Autodesk Inventor part; units mm, degrees
ref_plane "YZ Plane" through (0, 0, 0) normal (1, 0, 0) x (0, 1, 0)
ref_plane "XZ Plane" through (0, 0, 0) normal (0, 1, 0) x (-1, 0, 0)
ref_plane "XY Plane" through (0, 0, 0) normal (0, 0, 1) x (1, 0, 0)
sketch "Sketch1" plane through (0, 0, 0) normal (0, 1, 0) x (-1, 0, 0)
  line L0 (140, 210) -> (-140, 210)
  line L1 (-140, 210) -> (-140, -210)
  line L2 (-140, -210) -> (140, -210)
  line L3 (140, -210) -> (140, 210)
  line L4 (140, 210) -> (-140, -210) construction
  line L5 (-140, 210) -> (140, -210) construction
  point P0 (0, 0)
  dimension "d0" = 280
  dimension "d1" = 420
extrude "Extrusion1" add sketch "Sketch1" along normal blind 6
sketch "Sketch2" plane through (0, 6, 0) normal (0, 1, 0) x (1, 0, 0)
  circle A0 centre (105, -175) radius 14
  line L0 (-140, -210) -> (140, -210)
  line L1 (140, -210) -> (140, 210)
  point P0 (0, 0)
  dimension "d4" = 28
  dimension "d5" = 35
  dimension "d6" = 35
extrude "Extrusion2" cut sketch "Sketch2" against normal blind 6
sketch "Sketch3" plane through (0, 6, 0) normal (0, 1, 0) x (1, 0, 0)
  circle A0 centre (135, -205) radius 1.75
  line L0 (-140, -210) -> (140, -210)
  line L1 (140, -210) -> (140, 210)
  circle A1 centre (75.5, -205) radius 1.75
  circle A2 centre (135, -145.5) radius 1.75
  circle A3 centre (75.5, -145.5) radius 1.75
  point P0 (0, 0)
  dimension "d15" = 3.5
  dimension "d16" = 5
  dimension "d17" = 5
  dimension "d18" = 3.5
  dimension "d19" = 5
  dimension "d20" = 59.5
  dimension "d21" = 3.5
  dimension "d22" = 5
  dimension "d23" = 59.5
  dimension "d24" = 3.5
  dimension "d25" = 59.5
  dimension "d26" = 59.5
pattern_linear "Rectangular Pattern1" count 6 spacing 70 along (0, 0, -1) count 4 spacing 70 along (-1, 0, 0) of "Extrusion2"
sketch "Sketch4" plane through (0, 6, 0) normal (0, 1, 0) x (1, 0, 0)
  line L0 (140, -210) -> (140, 210)
  line L1 (140, -25) -> (134, -25)
  line L2 (134, -25) -> (134, 25)
  line L3 (134, 25) -> (140, 25)
  line L4 (140, 25) -> (140, -25)
  line L5 (0, -210) -> (0, 210) construction
  line L6 (140, -165) -> (134, -165)
  line L7 (134, -165) -> (134, -115)
  line L8 (134, -115) -> (140, -115)
  line L9 (140, -115) -> (140, -165)
  line L10 (-140, -210) -> (140, -210)
  line L11 (140, 115) -> (134, 115)
  line L12 (134, 115) -> (134, 165)
  line L13 (134, 165) -> (140, 165)
  line L14 (140, 165) -> (140, 115)
  line L15 (140, 210) -> (-140, 210)
  line L16 (-140, -25) -> (-134, -25)
  line L17 (-134, -25) -> (-134, 25)
  line L18 (-134, 25) -> (-140, 25)
  line L19 (-140, 25) -> (-140, -25)
  line L20 (-140, -165) -> (-134, -165)
  line L21 (-134, -165) -> (-134, -115)
  line L22 (-134, -115) -> (-140, -115)
  line L23 (-140, -115) -> (-140, -165)
  line L24 (-140, 115) -> (-134, 115)
  line L25 (-134, 115) -> (-134, 165)
  line L26 (-134, 165) -> (-140, 165)
  line L27 (-140, 165) -> (-140, 115)
  line L28 (-95, -210) -> (-45, -210)
  line L29 (-45, -210) -> (-45, -204)
  line L30 (-45, -204) -> (-95, -204)
  line L31 (-95, -204) -> (-95, -210)
  line L32 (-140, 210) -> (-140, -210)
  line L33 (45, -210) -> (95, -210)
  line L34 (95, -210) -> (95, -204)
  line L35 (95, -204) -> (45, -204)
  line L36 (45, -204) -> (45, -210)
  line L37 (-140, 0) -> (140, 0) construction
  line L38 (-95, 210) -> (-45, 210)
  line L39 (-45, 210) -> (-45, 204)
  line L40 (-45, 204) -> (-95, 204)
  line L41 (-95, 204) -> (-95, 210)
  line L42 (45, 210) -> (95, 210)
  line L43 (95, 210) -> (95, 204)
  line L44 (95, 204) -> (45, 204)
  line L45 (45, 204) -> (45, 210)
  point P0 (0, 0)
  dimension "d35" = 6
  dimension "d36" = 50
  dimension "d37" = 6
  dimension "d38" = 50
  dimension "d39" = 45
  dimension "d40" = 6
  dimension "d41" = 50
  dimension "d42" = 45
  dimension "d43" = 50
  dimension "d44" = 6
  dimension "d45" = 45
  dimension "d46" = 50
  dimension "d47" = 6
  dimension "d48" = 45
extrude "Extrusion4" cut sketch "Sketch4" against normal blind 6 contours L6 L7 L8 L0 | L10 L36 L35 L34 | L1 L2 L3 L0 | L10 L31 L30 L29 | L11 L12 L13 L0 | L23 L22 L21 L20 | L43 L44 L45 L15 | L19 L18 L17 L16 | L39 L40 L41 L15 | L27 L26 L25 L24
equation "\"d17\" = d16"
equation "\"d19\" = d16"
equation "\"d22\" = d16"
equation "\"d23\" = d20"
equation "\"d25\" = d20"
equation "\"d26\" = d20"
properties part number "Base_modulos"
Read the model definition and answer for the solid it produces. Units are mm, in the model's axes. Coordinates: 2 decimals unless noted, no trailing zeros. Loops run counter-clockwise (first coordinate to the right, second up) from the corner with the lowest first, then second, coordinate; pieces in that order, holes last. Notation, with made-up numbers: (22.25, 63.25) - (70.25, 63.25) arc R37 ccw to (70.25, 102.25) - close; hole circle Ø5 at (-13.75, -36). An arc over 180 degrees is marked (long way). Answer in a Markdown table with one row per item.
Q1. The mould has two halves that part along X. Classify faces 1 (the cylindrical face through (103.18, 3.04, -118.88)), 2 (the flat face through (2, 0, 3)): pulls with the +X half, pulls with the -X half, needs draft (parallel to the pull), parting line crosses it, or undercut.
Here are the results:
| item | result |
|---|---|
| face 1 | undercut |
| face 2 | needs draft |
Q2. Straight lines are drawn through the part: line 1 along X through (y, z) = (2.15, -175); line 2 along X through (y, z) = (4.7, 47); line 3 along Z through (x, y) = (-60, 0.55). For each, find the intervals that lie inside material, in ascending order. Write a range as [from, to].
Here are the results:
| item | result |
|---|---|
| line 1 | x = [-140, -119], [-91, -49], [-21, 21], [49, 91], [119, 140] |
| line 2 | x = [-140, -112.21], [-97.79, -42.21], [-27.79, 27.79], [42.21, 97.79], [112.21, 140] |
| line 3 | z = [-204, 204] |
Q3. Find section C-C on x = -38.5. Write down the section's boundary in (y, z).
Here are the results:
| item | result |
|---|---|
| outline | (0, -210) - (6, -210) - (6, -188.56) - (0, -188.56) - close; (0, -161.44) - (6, -161.44) - (6, -118.56) - (0, -118.56) - close; (0, -91.44) - (6, -91.44) - (6, -48.56) - (0, -48.56) - close; (0, -21.44) - (6, -21.44) - (6, 21.44) - (0, 21.44) - close; (0, 48.56) - (6, 48.56) - (6, 91.44) - (0, 91.44) - close; (0, 118.56) - (6, 118.56) - (6, 161.44) - (0, 161.44) - close; (0, 188.56) - (6, 188.56) - (6, 210) - (0, 210) - close |
Q4. Given P1, Ø25, axis at x = 35, z = 35, coming from the -Y side; P2, Ø2, axis at x = -50.5, y = 4, coming from the -Z side; P3, Ø3, axis at y = 4, z = -147.5, coming from the -X side, each flat-ended and moving along its own axis, determine where each tip first touches the part or whether it passes through.
Here are the results:
| item | result |
|---|---|
| P1 | passes through |
| P2 | stops at z = -204 |
| P3 | stops at x = -134 |
Q5. Find section B-B on z = 35. Write down the section's boundary in (x, y), plus the area to 3 significant figures.
Here are the results:
| item | result |
|---|---|
| outline | (-140, 0) - (-119, 0) - (-119, 6) - (-140, 6) - close; (-91, 0) - (-49, 0) - (-49, 6) - (-91, 6) - close; (-21, 0) - (21, 0) - (21, 6) - (-21, 6) - close; (49, 0) - (91, 0) - (91, 6) - (49, 6) - close; (119, 0) - (140, 0) - (140, 6) - (119, 6) - close |
| area | 1,010 mm^2 |
Q6. Find section D-D on y = 1.75. Count the separate pieces of the cut face and the enclosed holes in it, plus the area to 3 significant figures.
Here are the results:
| item | result |
|---|---|
| separate pieces | 1 |
| enclosed holes | 24 |
| area | 99,800 mm^2 |
Q7. Find section A-A on x = -105. Write down the section's boundary in (y, z).
Here are the results:
| item | result |
|---|---|
| outline | (0, -210) - (6, -210) - (6, -189) - (0, -189) - close; (0, -161) - (6, -161) - (6, -119) - (0, -119) - close; (0, -91) - (6, -91) - (6, -49) - (0, -49) - close; (0, -21) - (6, -21) - (6, 21) - (0, 21) - close; (0, 49) - (6, 49) - (6, 91) - (0, 91) - close; (0, 119) - (6, 119) - (6, 161) - (0, 161) - close; (0, 189) - (6, 189) - (6, 210) - (0, 210) - close |
